```python
from build123d import *

# Parameters (mm, degrees)
SKETCH_1_R      = 0.36
SKETCH_1_R_2    = 0.865
EXTRUDE_1_DEPTH = 1.1
EXTRUDE_START   = 2
SKETCH_2_R      = 2.7200000000000006
SKETCH_2_R_2    = 1.95
EXTRUDE_2_DEPTH = 2
FILLET_1_R      = 0.2


with BuildPart() as part:
    # 草图1 → 凸台-拉伸1 (new body)
    # profile 1 of 3: a face of its own
    with BuildSketch(Plane.XY):
        with BuildLine():
            Line((-2.0989282979654043, 1.7299999999999998), (-6.029999999999999, 1.7299999999999998))
            ThreePointArc((-6.029999999999999, 1.7299999999999995), (-7.759999999999999, -1.2e-16), (-6.029999999999999, -1.73))
            Line((-6.029999999999999, -1.7299999999999998), (-2.098928297965404, -1.7299999999999998))
            ThreePointArc((-2.0989282979654083, -1.7300000000000109), (-2.7200000000000006, 3.3e-16), (-2.098928297965408, 1.7300000000000115))
        make_face()
        with Locations((-6.029999999999999, 0)):
            Circle(SKETCH_1_R, mode=Mode.SUBTRACT)
        with Locations((-4.590000000000001, 0)):
            Circle(SKETCH_1_R, mode=Mode.SUBTRACT)
    # profile 2 of 3: a face of its own
    with BuildSketch(Plane.XY):
        with BuildLine():
            Line((0, 1.7299999999999998), (-2.0989282979654043, 1.7299999999999998))
            ThreePointArc((-2.098928297965408, 1.7300000000000115), (-2.7200000000000006, 3.3e-16), (-2.0989282979654083, -1.7300000000000109))
            Line((-2.098928297965404, -1.7299999999999998), (0, -1.7299999999999998))
            ThreePointArc((0, -1.7299999999999995), (1.7299999999999998, 1e-17), (2.1e-16, 1.73))
        make_face()
        Circle(SKETCH_1_R_2, mode=Mode.SUBTRACT)
    # profile 3 of 3: a face of its own
    with BuildSketch(Plane.XY):
        with BuildLine():
            ThreePointArc((2.7200000000000006, 0), (0.9190525092545292, 2.5600278289958016), (-2.098928297965408, 1.7300000000000115))
            Line((-2.0989282979654043, 1.7299999999999998), (0, 1.7299999999999998))
            ThreePointArc((2.1e-16, 1.73), (1.7299999999999998, 1e-17), (0, -1.7299999999999995))
            Line((0, -1.7299999999999998), (-2.098928297965404, -1.7299999999999998))
            ThreePointArc((-2.0989282979654083, -1.7300000000000109), (0.9190525092545296, -2.5600278289958016), (2.7200000000000006, -6.7e-16))
        make_face()
    extrude(amount=EXTRUDE_1_DEPTH)

    # 草图2 → 凸台-拉伸2 (add)
    with BuildSketch(Plane(origin=(0, 0, 0), x_dir=(-1, 0, 0), z_dir=(0, 0, -1)).offset(EXTRUDE_START)):
        Circle(SKETCH_2_R)
        Circle(SKETCH_2_R_2, mode=Mode.SUBTRACT)
    extrude(amount=-EXTRUDE_2_DEPTH)

    # 圆角1
    fillet_1_edges = [part.edges().sort_by_distance(p)[0] for p in [
        (2.7200000000000015, 1e-15, 1.1),
    ]]
    fillet(fillet_1_edges, radius=FILLET_1_R)


solid = part.part
```
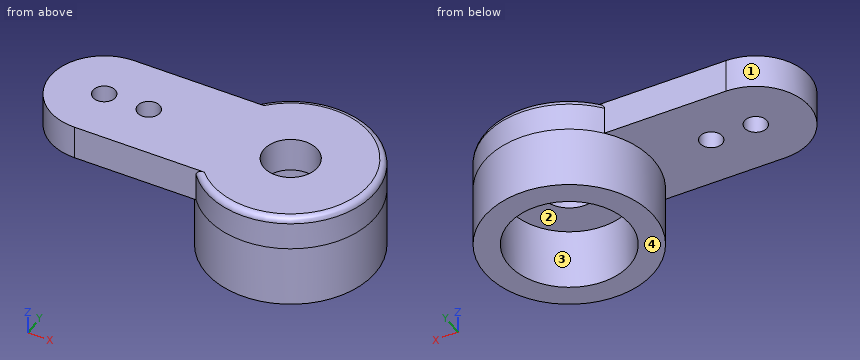
Geometry: final body of the model. Coordinates: model frame, mm. Face numbers are marked on the shaded views. Give positions to 0.01 mm unless a question says otherwise; leave off trailing zeros. Write each loop counter-clockwise with the first axis right and the second up, starting at its lowest first coordinate (ties: lowest second). Pieces come first, ordered by that corner, then holes.
1. Draft query along Y for the marked faces 1, 2, 3 and 4. Return one class per face: released by +Y, released by -Y, zero draft, split by the parting line, or undercut.
2. Line query: probe 1 along Z at (x, y) = (-1, -0.45); probe 2 along Y at (x, z) = (-4.59, 0.4); probe 3 along Y at (x, z) = (-1.75, -0.05). Output: solid intervals per line, ascending.
3. Section query B-B, the plane z = 0.7. Return loops of the section in (x, y) (3 decimals).
4. Section query A-A, the plane x = 0. Return loops of the section in (y, z) (3 decimals).
5. Pin query (flat end, axial travel): P1, Ø0.9, axis at x = -4, z = 0.5, coming from the +Y side; P2, Ø1.2, axis at x = -3, z = 0.5, coming from the -Y side; P3, Ø2, axis at x = 0, y = 0, coming from the +Z side; P4, Ø1, axis at x = -5.5, y = 0.5, coming from the -Z side. Return the tip coordinate at first contact, or that it passes through.
6. Section query C-C, the plane y = 0. Return loops of the section in (x, z) (3 decimals).
7. Section query D-D, the plane z = -0.7. Return loops of the section in (x, y), then the cut area to 3 significant figures.
Computed:
1. face 1: split by the parting line
1. face 2: undercut
1. face 3: undercut
1. face 4: zero draft
2. probe 1: z = 0 to 1.1
2. probe 2: y = -1.73 to -0.36, 0.36 to 1.73
2. probe 3: y = -2.08 to -0.86, 0.86 to 2.08
3. outline: (-6.03, -1.73) - (-2.099, -1.73) arc R2.72 ccw (long way) to (-2.099, 1.73) - (-6.03, 1.73) arc R1.73 ccw to start; hole circle Ø0.72 at (-6.03, 0); hole circle Ø0.72 at (-4.59, 0); hole circle Ø1.73 at (0, 0)
4. outline: (-2.72, -2) - (-1.95, -2) - (-1.95, 0) - (-0.865, 0) - (-0.865, 1.1) - (-2.52, 1.1) arc R0.2 ccw to (-2.72, 0.9) - close; (0.865, 0) - (1.95, 0) - (1.95, -2) - (2.72, -2) - (2.72, 0.9) arc R0.2 ccw to (2.52, 1.1) - (0.865, 1.1) - close
5. P1: stops at y = 1.73
5. P2: stops at y = -1.73
5. P3: stops at z = 1.1
5. P4: stops at z = 0
6. outline: (-7.76, 0) - (-6.39, 0) - (-6.39, 1.1) - (-7.76, 1.1) - close; (-5.67, 0) - (-4.95, 0) - (-4.95, 1.1) - (-5.67, 1.1) - close; (-4.23, 0) - (-2.72, 0) - (-2.72, -2) - (-1.95, -2) - (-1.95, 0) - (-0.865, 0) - (-0.865, 1.1) - (-4.23, 1.1) - close; (0.865, 0) - (1.95, 0) - (1.95, -2) - (2.72, -2) - (2.72, 0.9) arc R0.2 ccw to (2.52, 1.1) - (0.865, 1.1) - close
7. outline: circle Ø5.44 at (0, 0); hole circle Ø3.9 at (0, 0)
7. area: 11.3 mm2
